Can you work these out from the model? Positions are in its coordinate system, mm. Coordinates: 2 decimals unless noted, no trailing zeros. Order: outer loops, then holes, each group sorted by start corner. A loop starts at its lowest first (then second) coordinate and runs counter-clockwise, first axis right, second up. Notation, with made-up numbers: (-8, 42.25) -> (24, 42.25) arc R36 ccw to (24, 76.25) -> close; hole circle Ø4 at (-33, 35.5). An arc over 180 degrees is marked (long way). Answer as a JSON object with one key per item and string values. Group by question number.
(1) I want a section at A-A, the plane z = 0.7. State how many separate pieces and enclosed holes the cut face has, plus the area to 3 significant figures.
(2) I want a section at B-B, the plane x = 637. List the corners of the cut face in (y, z) for me.
(3) For pin 1 (1 mm diameter, centred on x = 593.5, z = 0, fed in from +Y), with a flat end and sliding along its axis, tell me the tip position at first contact or that it passes through.
(4) I need wall thicknesses on line 1 (Y direction, x = 500, z = 1.5); line 2 (X direction, y = 359, z = 0.25); line 3 (Y direction, x = 666, z = 0.85). Which ranges of each line are inside material? Lowest first, please.
(5) I want a section at C-C, the plane y = 479. List the corners of the cut face in (x, z) for me, plus the area to 3 significant figures.
Autodesk Inventor part; units mm, degrees
ref_plane "YZ Plane" through (0, 0, 0) normal (1, 0, 0) x (0, 1, 0)
ref_plane "XZ Plane" through (0, 0, 0) normal (0, 1, 0) x (-1, 0, 0)
ref_plane "XY Plane" through (0, 0, 0) normal (0, 0, 1) x (1, 0, 0)
sketch "Эскиз1" plane through (0, 0, 0) normal (0, 0, 1) x (1, 0, 0)
  line L0 (0, 0) -> (810, 0)
  line L1 (810, 0) -> (810, 300)
  line L2 (810, 300) -> (0, 300)
  line L3 (0, 300) -> (0, 0)
  line L4 (280, 300) -> (530, 300) construction
  line L5 (530, 300) -> (530, 0) construction
  line L6 (530, 0) -> (280, 0) construction
  line L7 (280, 0) -> (280, 300) construction
  line L8 (280, 300) -> (530, 300)
  line L9 (530, 300) -> (530, 580)
  line L10 (530, 580) -> (280, 580)
  line L11 (280, 580) -> (280, 300)
  line L12 (0, 300) -> (45, 345)
  line L13 (45, 345) -> (235, 345)
  line L14 (235, 345) -> (280, 300)
  line L15 (530, 300) -> (575, 345)
  line L16 (575, 345) -> (765, 345)
  line L17 (765, 345) -> (810, 300)
  dimension "d0" = 300
  dimension "d1" = 810
  dimension "d2" = 250
  dimension "d3" = 280
  dimension "d4" = 280
  dimension "d5" = 280
  dimension "d6" = 45
extrude "Выдавливание1" add sketch "Эскиз1" along normal blind 2
sketch "Эскиз2" plane through (0, 0, 2) normal (0, 0, 1) x (1, 0, 0)
  line L0 (45, 345) -> (0, 300)
  line L1 (0, 300) -> (0, 0)
  line L2 (0, 0) -> (810, 0)
  line L3 (810, 0) -> (810, 300)
  line L4 (810, 300) -> (765, 345)
  line L5 (765, 345) -> (575, 345)
  line L6 (575, 345) -> (530, 300)
  line L7 (530, 300) -> (530, 580)
  line L8 (530, 580) -> (280, 580)
  line L9 (280, 580) -> (280, 300)
  line L10 (280, 300) -> (235, 345)
  line L11 (235, 345) -> (45, 345)
  line L12 (280, 300) -> (530, 300) construction
  line L13 (530, 300) -> (530, 0) construction
  line L14 (530, 0) -> (280, 0) construction
  line L15 (280, 0) -> (280, 300) construction
  line L16 (530, 300) -> (530, 580) construction
  circle A0 centre (310, 270) radius 1.5
  circle A1 centre (500, 270) radius 1.5
  circle A2 centre (310, 30) radius 1.5
  circle A3 centre (500, 30) radius 1.5
  line L17 (500, 270) -> (310, 270) construction
  line L18 (310, 270) -> (310, 30) construction
  line L19 (310, 30) -> (500, 30) construction
  line L20 (500, 30) -> (500, 270) construction
  line L21 (290, 162.5) -> (300, 162.5)
  line L22 (300, 162.5) -> (300, 137.5)
  line L23 (300, 137.5) -> (290, 137.5)
  line L24 (290, 137.5) -> (290, 162.5)
  line L25 (510, 162.5) -> (520, 162.5)
  line L26 (520, 162.5) -> (520, 137.5)
  line L27 (520, 137.5) -> (510, 137.5)
  line L28 (510, 137.5) -> (510, 162.5)
  line L29 (280, 150) -> (530, 150) construction
  line L30 (390, 20) -> (420, 20)
  line L31 (420, 20) -> (420, 10)
  line L32 (420, 10) -> (390, 10)
  line L33 (390, 10) -> (390, 20)
  line L34 (405, 300) -> (405, 0) construction
  line L35 (0, 0) -> (810, 0) construction
  line L36 (325, 10) -> (295, 10)
  line L37 (295, 10) -> (295, 20)
  line L38 (295, 20) -> (325, 20)
  line L39 (325, 20) -> (325, 10)
  line L40 (485, 10) -> (515, 10)
  line L41 (515, 10) -> (515, 20)
  line L42 (515, 20) -> (485, 20)
  line L43 (485, 20) -> (485, 10)
  point P0 (290, 150)
  point P1 (510, 150)
  point P2 (405, 20)
  dimension "d9" = 3
  dimension "d10" = 30
  dimension "d11" = 30
  dimension "d12" = 30
  dimension "d13" = 30
  dimension "d16" = 10
  dimension "d17" = 25
  dimension "d18" = 10
  dimension "d19" = 10
  dimension "d20" = 10
  dimension "d21" = 30
  dimension "d22" = 10
  dimension "d23" = 30
  dimension "d24" = 15
extrude "Выдавливание2" cut sketch "Эскиз2" against normal through all contours A0 | A1 | A2 | A3 | L21 L22 L23 L24 | L25 L26 L27 L28 | L30 L31 L32 L33 | L36 L37 L38 L39 | L43 L42 L41 L40
properties part number "head_without_face"
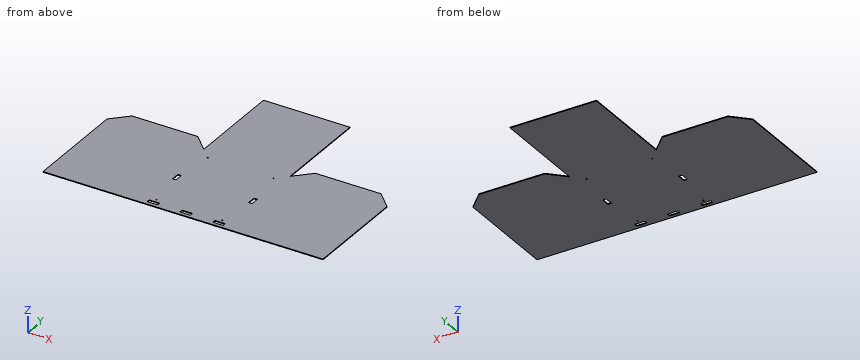
Computed values:
{
 "1": {"separate pieces": "1", "enclosed holes": "9", "area": "333,000 mm2"},
 "2": {"outline": "(0, 0) -> (345, 0) -> (345, 2) -> (0, 2) -> close"},
 "3": {"pin 1": "stops at y = 345"},
 "4": {"line 1": "y = 0 to 10, 20 to 28.5, 31.5 to 268.5, 271.5 to 580", "line 2": "x = 280 to 530", "line 3": "y = 0 to 345"},
 "5": {"outline": "(280, 0) -> (530, 0) -> (530, 2) -> (280, 2) -> close", "area": "500 mm2"}
}
